from build123d import *

# Parameters (mm, degrees)
F0_W     = 32
F0_H     = 8
F0_R     = 2.4
F0_R_2   = 1.6
F1_DEPTH = 3.2
F2_T     = -1.6
F3_DEPTH = 1.6
F4_START = 3.2
F4_DEPTH = 1.6


with BuildPart() as f1:
    # F0 (on Top) → F1 (new body)
    with BuildSketch(Plane.XY):
        Rectangle(F0_W, F0_H)
        with Locations((-12, 0)):
            Circle(F0_R, mode=Mode.SUBTRACT)
        with BuildLine():
            ThreePointArc((-6.4, 0), (-8, -1.6), (-9.6, 0))
            ThreePointArc((-9.6, 0), (-8, 1.6), (-6.4, 0))
        make_face(mode=Mode.SUBTRACT)
        with BuildLine():
            ThreePointArc((-1.6, 0), (-4, -2.4), (-6.4, 0))
            ThreePointArc((-6.4, 0), (-4, 2.4), (-1.6, 0))
        make_face(mode=Mode.SUBTRACT)
        with BuildLine():
            ThreePointArc((1.6, 0), (0, -1.6), (-1.6, 0))
            ThreePointArc((-1.6, 0), (0, 1.6), (1.6, 0))
        make_face(mode=Mode.SUBTRACT)
        with BuildLine():
            ThreePointArc((6.4, 0), (4, -2.4), (1.6, 0))
            ThreePointArc((1.6, 0), (4, 2.4), (6.4, 0))
        make_face(mode=Mode.SUBTRACT)
        with BuildLine():
            ThreePointArc((9.6, 0), (8, -1.6), (6.4, 0))
            ThreePointArc((6.4, 0), (8, 1.6), (9.6, 0))
        make_face(mode=Mode.SUBTRACT)
        with BuildLine():
            ThreePointArc((14.4, 0), (12, -2.4), (9.6, 0))
            ThreePointArc((9.6, 0), (12, 2.4), (14.4, 0))
        make_face(mode=Mode.SUBTRACT)
        with Locations((-12, 0)):
            Circle(F0_R)
        with Locations((-12, 0)):
            Circle(F0_R_2, mode=Mode.SUBTRACT)
        with BuildLine():
            ThreePointArc((-1.6, 0), (-4, 2.4), (-6.4, 0))
            ThreePointArc((-6.4, 0), (-4, -2.4), (-1.6, 0))
        make_face()
        with Locations((-4, 0)):
            Circle(F0_R_2, mode=Mode.SUBTRACT)
        with BuildLine():
            ThreePointArc((6.4, 0), (4, 2.4), (1.6, 0))
            ThreePointArc((1.6, 0), (4, -2.4), (6.4, 0))
        make_face()
        with Locations((4, 0)):
            Circle(F0_R_2, mode=Mode.SUBTRACT)
        with BuildLine():
            ThreePointArc((14.4, 0), (12, 2.4), (9.6, 0))
            ThreePointArc((9.6, 0), (12, -2.4), (14.4, 0))
        make_face()
        with Locations((12, 0)):
            Circle(F0_R_2, mode=Mode.SUBTRACT)
        with Locations((-12, 0)):
            Circle(F0_R_2)
        with BuildLine():
            ThreePointArc((-6.4, 0), (-8, 1.6), (-9.6, 0))
            ThreePointArc((-9.6, 0), (-8, -1.6), (-6.4, 0))
        make_face()
        with Locations((-4, 0)):
            Circle(F0_R_2)
        with BuildLine():
            ThreePointArc((1.6, 0), (0, 1.6), (-1.6, 0))
            ThreePointArc((-1.6, 0), (0, -1.6), (1.6, 0))
        make_face()
        with Locations((4, 0)):
            Circle(F0_R_2)
        with BuildLine():
            ThreePointArc((9.6, 0), (8, 1.6), (6.4, 0))
            ThreePointArc((6.4, 0), (8, -1.6), (9.6, 0))
        make_face()
        with Locations((12, 0)):
            Circle(F0_R_2)
    extrude(amount=F1_DEPTH)

    # F2
    f2_openings = [f1.faces().sort_by_distance(p)[0] for p in [
        (0, 0, 0),
    ]]
    offset(amount=F2_T, openings=f2_openings)

    # F0 (on Top) → F3 (join, through all)
    with BuildSketch(Plane.XY):
        with BuildLine():
            ThreePointArc((-6.4, 0), (-8, 1.6), (-9.6, 0))
            ThreePointArc((-9.6, 0), (-8, -1.6), (-6.4, 0))
        make_face()
        with BuildLine():
            ThreePointArc((1.6, 0), (0, 1.6), (-1.6, 0))
            ThreePointArc((-1.6, 0), (0, -1.6), (1.6, 0))
        make_face()
        with BuildLine():
            ThreePointArc((9.6, 0), (8, 1.6), (6.4, 0))
            ThreePointArc((6.4, 0), (8, -1.6), (9.6, 0))
        make_face()
    extrude(amount=F3_DEPTH)

    # F0 (on Top) → F4 (join)
    with BuildSketch(Plane.XY.offset(F4_START)):
        with Locations((-12, 0)):
            Circle(F0_R)
        with Locations((-12, 0)):
            Circle(F0_R_2, mode=Mode.SUBTRACT)
        with BuildLine():
            ThreePointArc((-1.6, 0), (-4, 2.4), (-6.4, 0))
            ThreePointArc((-6.4, 0), (-4, -2.4), (-1.6, 0))
        make_face()
        with Locations((-4, 0)):
            Circle(F0_R_2, mode=Mode.SUBTRACT)
        with BuildLine():
            ThreePointArc((6.4, 0), (4, 2.4), (1.6, 0))
            ThreePointArc((1.6, 0), (4, -2.4), (6.4, 0))
        make_face()
        with Locations((4, 0)):
            Circle(F0_R_2, mode=Mode.SUBTRACT)
        with BuildLine():
            ThreePointArc((14.4, 0), (12, 2.4), (9.6, 0))
            ThreePointArc((9.6, 0), (12, -2.4), (14.4, 0))
        make_face()
        with Locations((12, 0)):
            Circle(F0_R_2, mode=Mode.SUBTRACT)
        with Locations((-12, 0)):
            Circle(F0_R_2)
        with Locations((-4, 0)):
            Circle(F0_R_2)
        with Locations((4, 0)):
            Circle(F0_R_2)
        with Locations((12, 0)):
            Circle(F0_R_2)
    extrude(amount=F4_DEPTH)


solid = f1.part
Verification items for the finished model (mm, model axes). A direction names the side the tool comes from. Round coordinates to 2 decimals unless told otherwise and drop trailing zeros. Order: outer loops, then holes, each group sorted by start corner. A loop starts at its lowest first (then second) coordinate and runs counter-clockwise, first axis right, second up.
1. Go/stop test with a flat-tipped pin: P1, Ø1, axis at y = -1.5, z = 4, coming from the +X side. Record where the tip stops, or that it passes through.
Final values:
P1: stops at x = 14.18
2. Access from +Z, -Z, +X, -X, +Y, -Y to the whole of each face (thin tool, end or side, straight path). Record for faces 1 (the cylindrical face through (-6.4, -0.07, 0.79)), 2 (the flat face through (0, 0, 3.2)), 3 (the flat face through (12, 0, 4.8)).
Final values:
face 1: -Z
face 2: +Z
face 3: +Z, +X, -X, +Y, -Y
3. Release check for a two-part mould opening along Y. For faces 4 (the flat face through (0, -2.4, 1)), 5 (the flat face through (0, 2, 1.6)), 6 (the flat face through (-8, 0, 0)), 7 (the cylindrical face through (1.783, 0.919, 3.989)) record: +Y half, -Y half, draft (parallel to the pull), parting line (faces both ways), or undercut.
Final values:
face 4: undercut
face 5: undercut
face 6: draft
face 7: parting line
4. Section check B-B on x = -8. Record the cut outline in (y, z).
Final values:
outline: (-4, 0) - (-2.4, 0) - (-2.4, 1.6) - (-1.6, 1.6) - (-1.6, 0) - (1.6, 0) - (1.6, 1.6) - (2.4, 1.6) - (2.4, 0) - (4, 0) - (4, 3.2) - (-4, 3.2) - close
5. Thickness scan on L1, parallel to Y at x = -14, z = 0.3; L2, parallel to Z at x = 1.5, y = -0.25; L3, parallel to X at y = -2, z = 3.25. Record the ranges inside material, lowest first.
Final values:
L1: y = -4 to -2.4, 2.4 to 4
L2: z = 0 to 3.2
L3: x = -13.33 to -10.67, -5.33 to -2.67, 2.67 to 5.33, 10.67 to 13.33
6. Section check A-A on z = 3.8. Record the cut outline in (x, y).
Final values:
outline: circle Ø4.8 at (-12, 0); circle Ø4.8 at (-4, 0); circle Ø4.8 at (4, 0); circle Ø4.8 at (12, 0)
7. Section check C-C on x = 5.5. Record the cut outline in (y, z).
Final values:
outline: (-4, 0) - (-2.4, 0) - (-2.4, 1.6) - (2.4, 1.6) - (2.4, 0) - (4, 0) - (4, 3.2) - (1.87, 3.2) - (1.87, 4.8) - (-1.87, 4.8) - (-1.87, 3.2) - (-4, 3.2) - close
